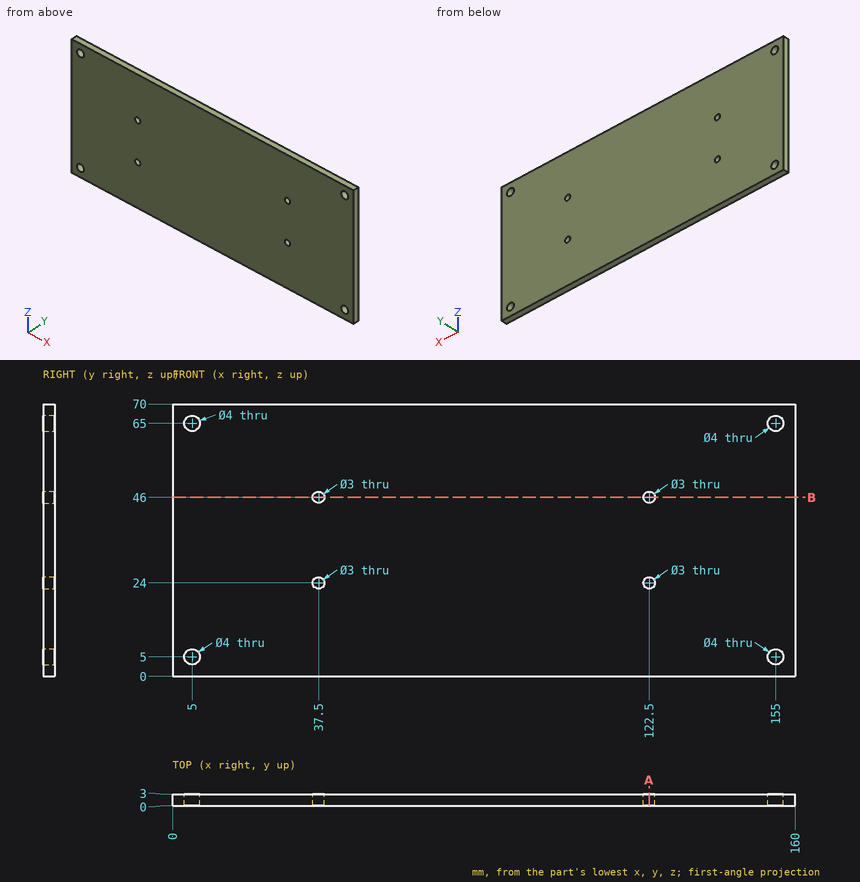
Geometry: see drawing. Coordinates: mm, zero at the bounding-box minimum. Coordinates: 2 decimals unless noted, no trailing zeros. Write each loop counter-clockwise with the first axis right and the second up, starting at its lowest first coordinate (ties: lowest second). Pieces come first, ordered by that corner, then holes.
1) Section B-B on z = 46. Output: boundary loops of the cut face in (x, y).
2) Pin query (flat end, axial travel): pin 1 Ø5 at (x, z) = (98.5, 33.5) entering from -Y. Return the tip coordinate at first contact, or that it passes through.
3) Material intervals for line 1 along Z through (x, y) = (155, 1.9); line 2 along X through (y, z) = (2.2, 5); line 3 along Z through (x, y) = (122.5, 1.05), sorted ascending.
4) Section A-A on x = 122.5. Output: boundary loops of the cut face in (y, z).
Check result:
1. outline: (0, 0) - (36, 0) - (36, 3) - (0, 3) - close; (39, 0) - (121, 0) - (121, 3) - (39, 3) - close; (124, 0) - (160, 0) - (160, 3) - (124, 3) - close
2. pin 1: stops at y = 0
3. line 1: z = 0 to 3, 7 to 63, 67 to 70
3. line 2: x = 0 to 3, 7 to 153, 157 to 160
3. line 3: z = 0 to 22.5, 25.5 to 44.5, 47.5 to 70
4. outline: (0, 0) - (3, 0) - (3, 22.5) - (0, 22.5) - close; (0, 25.5) - (3, 25.5) - (3, 44.5) - (0, 44.5) - close; (0, 47.5) - (3, 47.5) - (3, 70) - (0, 70) - close
